Here's how the part is built. I have some questions about the finished solid (model axes, mm). Face numbers are marked on the shaded views. A direction names the side the tool comes from. Give positions to 0.01 mm unless a question says otherwise; leave off trailing zeros. Loops run counter-clockwise (first coordinate to the right, second up) from the corner with the lowest first, then second, coordinate; pieces in that order, holes last. Notation, with made-up numbers: M 86.5,79 L 138.5,79 A9 ccw 138.5,92 Z; hole C -39.75,28 d2. An arc over 180 degrees is marked long. Write item = value, one per line. Start each with the question number.
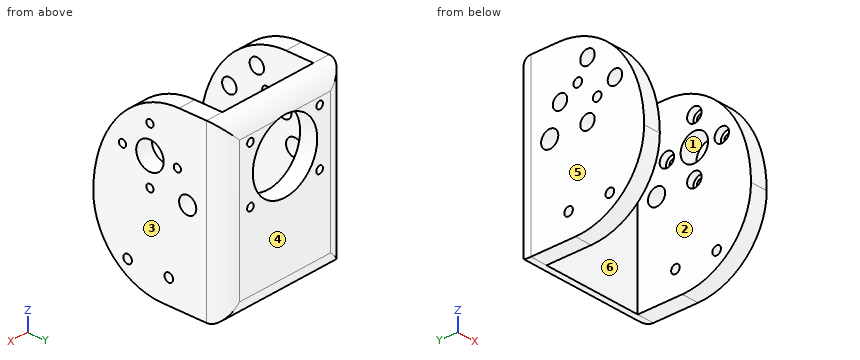
```python
from build123d import *

# Parameters (mm, degrees)
SKETCH1_W               = 30
SKETCH1_H               = 33
SKETCH1_R               = 1.05
SKETCH1_R_2             = 4
BOSS_EXTRUDE1_DEPTH     = 5
SKETCH2_W               = 39
SKETCH2_H               = 30
SKETCH2_R               = 10.25
SKETCH2_R_2             = 1.05
BOSS_EXTRUDE2_DEPTH     = 5
SKETCH3_W               = 30
SKETCH3_H               = 38
SKETCH3_R               = 1.25
BOSS_EXTRUDE3_DEPTH     = 5
BOSS_EXTRUDE5_DEPTH     = 20
SKETCH5_R               = 1.25
CUT_EXTRUDE1_DEPTH      = 57.641415943
SKETCH7_R               = 2.5
CUT_EXTRUDE2_DEPTH      = 57.641415943
FILLET1_SIZE            = 25
FILLET1_SIZE_2          = 30
FILLET2_R               = 20
FILLET3_START           = -34
FILLET3_DEPTH           = 39
FILLET3_START_2         = -36
FILLET3_2_DEPTH         = 52
CUT_EXTRUDE3_DEPTH      = 54.322134411
CUT_EXTRUDE3_DEPTH_BACK = 2
SKETCH8_R               = 2.1


with BuildPart() as part:
    # Sketch1 → Boss-Extrude1 (new body)
    with BuildSketch(Plane(origin=(0, 0, 0), x_dir=(0, 0, -1), z_dir=(1, 0, 0))):
        Rectangle(SKETCH1_W, SKETCH1_H)
        with Locations((0, 8)):
            Circle(SKETCH1_R, mode=Mode.SUBTRACT)
        with Locations((8, 0)):
            Circle(SKETCH1_R, mode=Mode.SUBTRACT)
        with Locations((0, -8)):
            Circle(SKETCH1_R, mode=Mode.SUBTRACT)
        with Locations((-8, 0)):
            Circle(SKETCH1_R, mode=Mode.SUBTRACT)
        Circle(SKETCH1_R_2, mode=Mode.SUBTRACT)
    extrude(amount=BOSS_EXTRUDE1_DEPTH)

    # Sketch2 → Boss-Extrude2 (add)
    with BuildSketch(Plane(origin=(0, 16.5, 0), x_dir=(1, 0, 0), z_dir=(0, 1, 0))):
        with Locations((-14.5, 0)):
            Rectangle(SKETCH2_W, SKETCH2_H)
        with Locations(Location((-14.5, 0, 0), (0, 0, 270))):
            Circle(SKETCH2_R, mode=Mode.SUBTRACT)
        with Locations(Location((-25.5, 8, 0), (0, 0, 270))):
            Circle(SKETCH2_R_2, mode=Mode.SUBTRACT)
        with Locations(Location((-3.5, 8, 0), (0, 0, 270))):
            Circle(SKETCH2_R_2, mode=Mode.SUBTRACT)
        with Locations(Location((-3.5, -8, 0), (0, 0, 270))):
            Circle(SKETCH2_R_2, mode=Mode.SUBTRACT)
        with Locations(Location((-25.5, -8, 0), (0, 0, 270))):
            Circle(SKETCH2_R_2, mode=Mode.SUBTRACT)
    extrude(amount=BOSS_EXTRUDE2_DEPTH)

    # Sketch3 → Boss-Extrude3 (add)
    with BuildSketch(Plane.ZY.offset(34)):
        with Locations((0, 2.5)):
            Rectangle(SKETCH3_W, SKETCH3_H)
        with Locations((2.828427125, 2.828427125)):
            Circle(SKETCH3_R, mode=Mode.SUBTRACT)
        with Locations((-2.828427125, -2.828427125)):
            Circle(SKETCH3_R, mode=Mode.SUBTRACT)
    extrude(amount=-BOSS_EXTRUDE3_DEPTH)

    # Sketch6 → Boss-Extrude5 (add)
    with BuildSketch(Plane(origin=(0, 0, -15), x_dir=(-1, 0, 0), z_dir=(0, 0, -1))):
        Polygon((0, 16.5), (29, 16.5), (29, -16.5), (34, -16.5), (34, 21.5), (-5, 21.5), (-5, -16.5), (0, -16.5), align=None)
    extrude(amount=BOSS_EXTRUDE5_DEPTH)

    # Sketch5 → Cut-Extrude1 (cut, through all)
    with BuildSketch(Plane.ZY.offset(34)):
        with Locations((-28, -6.5)):
            Circle(SKETCH5_R)
        with Locations((-28, 5.5)):
            Circle(SKETCH5_R)
    extrude(amount=-CUT_EXTRUDE1_DEPTH, mode=Mode.SUBTRACT)

    # Sketch7 → Cut-Extrude2 (cut, through all)
    with BuildSketch(Plane.ZY.offset(34)):
        with Locations((-8, 11)):
            Circle(SKETCH7_R)
    extrude(amount=-CUT_EXTRUDE2_DEPTH, mode=Mode.SUBTRACT)

    # Fillet1
    # a fillet whose section is not a circle: 30, 25 mm, written as the material it takes off along each edge
    with BuildSketch(Plane(origin=(-109, -16.5, 15), x_dir=(0, 1, 0), z_dir=(1, 0, 0))) as fillet1_piece_1:
        with BuildLine():
            Bezier((FILLET1_SIZE, 0), (0, 0), (0, -FILLET1_SIZE_2), weights=[1, 0.707106781, 1])
            Line((0, -FILLET1_SIZE_2), (0, 0))
            Line((0, 0), (FILLET1_SIZE, 0))
        make_face()
    extrude(amount=155, mode=Mode.SUBTRACT)
    with BuildSketch(Plane(origin=(-75, -16.5, 15), x_dir=(0, 0, -1), z_dir=(1, 0, 0))) as fillet1_piece_2:
        with BuildLine():
            Bezier((FILLET1_SIZE_2, 0), (0, 0), (0, FILLET1_SIZE), weights=[1, 0.707106781, 1])
            Line((0, FILLET1_SIZE), (0, 0))
            Line((0, 0), (FILLET1_SIZE_2, 0))
        make_face()
    extrude(amount=155, mode=Mode.SUBTRACT)

    # Fillet2
    fillet2_edges = [part.edges().sort_by_distance(p)[0] for p in [
        (2.5, -16.5, -35),
        (-31.5, -16.5, -35),
    ]]
    fillet(fillet2_edges, radius=FILLET2_R - 0.0001)  # a hair under: the kernel refuses the full size

    # Fillet3: read off the stored shape, not the designer's step
    # Fillet3 outline → Fillet3 (cut)
    with BuildSketch(Plane.YZ.offset(FILLET3_START)):
        with BuildLine():
            Line((21.5, 15), (16.5, 15))
            ThreePointArc((16.5, 15), (20.035533906, 13.535533906), (21.5, 10))
            Line((21.5, 10), (21.5, 15))
        make_face()
        with BuildLine():
            Line((21.5, -35), (21.5, -30))
            ThreePointArc((21.5, -30), (20.035533906, -33.535533906), (16.5, -35))
            Line((16.5, -35), (21.5, -35))
        make_face()
    extrude(amount=FILLET3_DEPTH, mode=Mode.SUBTRACT)

    # Fillet3 2 outline → Fillet3 2 (cut)
    with BuildSketch(Plane.XY.offset(FILLET3_START_2)):
        with BuildLine():
            Line((-34, 21.5), (-34, 16.5))
            ThreePointArc((-34, 16.5), (-32.535533906, 20.035533906), (-29, 21.5))
            Line((-29, 21.5), (-34, 21.5))
        make_face()
        with BuildLine():
            Line((5, 21.5), (0, 21.5))
            ThreePointArc((0, 21.5), (3.535533906, 20.035533906), (5, 16.5))
            Line((5, 16.5), (5, 21.5))
        make_face()
    extrude(amount=FILLET3_2_DEPTH, mode=Mode.SUBTRACT)

    # Sketch8 → Cut-Extrude3 (cut, two sides: drawn at the far end of the back side and taken through both)
    with BuildSketch(Plane.ZY.offset(-CUT_EXTRUDE3_DEPTH_BACK)):
        with Locations(Location((0, 8, 0), (0, 0, 180))):
            Circle(SKETCH8_R)
        with Locations(Location((8, 0, 0), (0, 0, 180))):
            Circle(SKETCH8_R)
        with Locations(Location((0, -8, 0), (0, 0, 180))):
            Circle(SKETCH8_R)
        with Locations(Location((-8, 0, 0), (0, 0, 180))):
            Circle(SKETCH8_R)
    extrude(amount=CUT_EXTRUDE3_DEPTH + CUT_EXTRUDE3_DEPTH_BACK, mode=Mode.SUBTRACT)


solid = part.part
```
Q1. If we section it at B-B, the plane y = 19.5: List the corners of the cut face in (x, z) for me, then the cut area to 3 significant figures.
Q2. If we section it at D-D, the plane z = -28: List the corners of the cut face in (x, y) for me, then the cut area to 3 significant figures.
Q3. Will these pins go through, and if not, where does the flat tip stop? pin 1 (1.3 mm diameter, centred on y = 0, z = -8.5, fed in from -X); pin 2 (2 mm diameter, centred on y = 2.83, z = 2.83, fed in from -X); pin 3 (6 mm diameter, centred on x = -0.5, z = -10.5, fed in from -Y).
Q4. If I drill on line 1 along Y through (x, z) = (1, -9.5); line 2 along X through (y, z) = (14.5, -26.5); line 3 along Y through (x, z) = (3.6, 0), over which ranges is the centre line in solid material (lowest first)?
Q5. If we section it at C-C, the plane x = -17.5: List the corners of the cut face in (y, z) for me.
Q6. If we section it at A-A, the plane x = -25.5: List the corners of the cut face in (y, z) for me, then the cut area to 3 significant figures.
Q7. On a 3-axis mill with a long thin cutter (end or side, diameter ignored), from which of +Z, -Z, +X, -X, +Y, -Y can I reach the whole of each face in a straight line? I mean the marked faces 1, 2 and 3. Say none if no direction works.
Q8. We'd pull the mould along X, two halves only. Please class the marked faces 4, 5 and 6: pulls with the +X half, pulls with the -X half, needs draft (parallel to the pull), parting line crosses it, or undercut.
Resolved:
q1.outline = M -33,-34 L 4,-34 L 4,14 L -33,14 Z; hole C -25.5,-8 d2.1; hole C -25.5,8 d2.1; hole C -14.5,0 d20.5; hole C -3.5,-8 d2.1; hole C -3.5,8 d2.1
q1.area = 1,430 mm²
q2.outline = M -34,-11.7 L -29,-11.7 L -29,-7.75 L -34,-7.75 Z; M -34,-5.25 L -29,-5.25 L -29,4.25 L -34,4.25 Z; M -34,6.75 L -29,6.75 L -29,16.5 L 0,16.5 L 0,6.75 L 5,6.75 L 5,16.5 A5 ccw 0,21.5 L -29,21.5 A5 ccw -34,16.5 Z; M 0,-11.7 L 5,-11.7 L 5,-7.75 L 0,-7.75 Z; M 0,-5.25 L 5,-5.25 L 5,4.25 L 0,4.25 Z
q2.area = 416 mm²
q3.pin_1 = 2
q3.pin_2 = 0
q3.pin_3 = -16.47
q4.line_1 = -16.08 to -1.47, 1.47 to 9, 13 to 21.4
q4.line_2 = -34 to -29, 0 to 5
q4.line_3 = -13.15 to -9.05, -6.95 to -4, 4 to 6.95, 9.05 to 19.97
q5.outline = M 16.5,-35 A5 ccw 21.5,-30 L 21.5,-9.8 L 16.5,-9.8 Z; M 16.5,9.8 L 21.5,9.8 L 21.5,10 A5 ccw 16.5,15 Z
q6.outline = M 16.5,-35 A5 ccw 21.5,-30 L 21.5,-9.05 L 16.5,-9.05 Z; M 16.5,-6.95 L 21.5,-6.95 L 21.5,6.95 L 16.5,6.95 Z; M 16.5,9.05 L 21.5,9.05 L 21.5,10 A5 ccw 16.5,15 Z
q6.area = 218 mm²
q7.face_1 = +X
q7.face_2 = +Z, -Z, -Y
q7.face_3 = +Z, -Z, +X, +Y, -Y
q8.face_4 = needs draft
q8.face_5 = pulls with the -X half
q8.face_6 = undercut
